Design review of the part built by this model. Coordinates are the model's own, in mm. Coordinates: 2 decimals unless noted, no trailing zeros. Loops run counter-clockwise (first coordinate to the right, second up) from the corner with the lowest first, then second, coordinate; pieces in that order, holes last. Notation, with made-up numbers: (57, 25.25) -> (73, 25.25) arc R20 ccw to (73, 47.25) -> close; hole circle Ø5 at (80, -33). An arc over 180 degrees is marked (long way). Use a Markdown table: item, result. Add a question column.
Q1. Clearance check with flat-ended pins moving along their axes: pin 1 Ø3 at (x, z) = (-33.02, 37.338) entering from +Y; pin 2 Ø1.5 at (x, y) = (172.5, 3.5) entering from +Z; pin 3 Ø1.5 at (x, z) = (-10.5, 17.5) entering from -Y. State where each tip first meets the part, or that it passes through.
Q2. Take a section at B-B on y = 3.85. Count the separate pieces of the cut face and the enclosed holes in it, plus the area to 3 significant figures.
Q3. Take a section at A-A on z = 68.58. Write out the cut boundary in (x, y) (1 decimal), plus the area to 3 significant figures.
Q4. Take a section at C-C on x = 88. Write out the cut boundary in (y, z).
Q5. For probe 1 along X at (y, z) = (3.5, -44.45); probe 2 along Z at (x, y) = (17.78, 2.2); probe 3 along X at (y, z) = (1.35, 70), list the stretches that pass through material, from the lowest coordinate up.
from build123d import *

# Parameters (mm, degrees)
SKETCH1_R               = 22.225
SKETCH1_W               = 373.38
SKETCH1_H               = 127
BOSS_EXTRUDE1_DEPTH     = 5.07492
SKETCH1_5_R             = 6.2865
CUT_EXTRUDE1_DEPTH      = 208.664293845
CUT_EXTRUDE2_DEPTH      = 208.664293845
CUT_EXTRUDE2_DEPTH_BACK = 208.664293845
SKETCH1_7_R             = 3.048
SKETCH1_8_R             = 2.54
SKETCH1_8_R_2           = 3.175
CUT_EXTRUDE3_DEPTH      = 208.664293845


with BuildPart() as part:
    # Sketch1 → Boss-Extrude1 (new body)
    with BuildSketch(Plane(origin=(0, 0, 0), x_dir=(1, 0, 0), z_dir=(0, 1, 0))):
        with Locations((-123.19, -68.58)):
            Circle(SKETCH1_R)
        with Locations((123.19, -68.58)):
            Circle(SKETCH1_R)
        Rectangle(SKETCH1_W, SKETCH1_H)
    extrude(amount=BOSS_EXTRUDE1_DEPTH)

    # Sketch1<5> → Cut-Extrude1 (cut, through all)
    with BuildSketch(Plane(origin=(0, 0, 0), x_dir=(1, 0, 0), z_dir=(0, 1, 0))):
        with Locations(Location((-123.19, -68.58, 0), (0, 0, 90))):
            Circle(SKETCH1_5_R)
        with Locations(Location((123.19, -68.58, 0), (0, 0, 90))):
            Circle(SKETCH1_5_R)
    extrude(amount=CUT_EXTRUDE1_DEPTH, mode=Mode.SUBTRACT)

    # Sketch1<7> → Cut-Extrude2 (cut, two sides: drawn at the far end of the back side and taken through both)
    with BuildSketch(Plane(origin=(0, 0, 0), x_dir=(1, 0, 0), z_dir=(0, 1, 0)).offset(-CUT_EXTRUDE2_DEPTH_BACK)):
        with Locations(Location((-123.19, 44.45, 0), (0, 0, 90))):
            Circle(SKETCH1_7_R)
        with Locations(Location((123.19, 44.45, 0), (0, 0, 90))):
            Circle(SKETCH1_7_R)
    extrude(amount=CUT_EXTRUDE2_DEPTH + CUT_EXTRUDE2_DEPTH_BACK, mode=Mode.SUBTRACT)

    # Sketch1<8> → Cut-Extrude3 (cut, through all)
    with BuildSketch(Plane(origin=(0, 0, 0), x_dir=(1, 0, 0), z_dir=(0, 1, 0))):
        with Locations(Location((-33.02, -37.338, 0), (0, 0, 90))):
            Circle(SKETCH1_8_R)
        with Locations(Location((17.78, -37.338, 0), (0, 0, 90))):
            Circle(SKETCH1_8_R)
        with Locations(Location((0, -54.864, 0), (0, 0, 90))):
            Circle(SKETCH1_8_R_2)
    extrude(amount=CUT_EXTRUDE3_DEPTH, mode=Mode.SUBTRACT)


solid = part.part
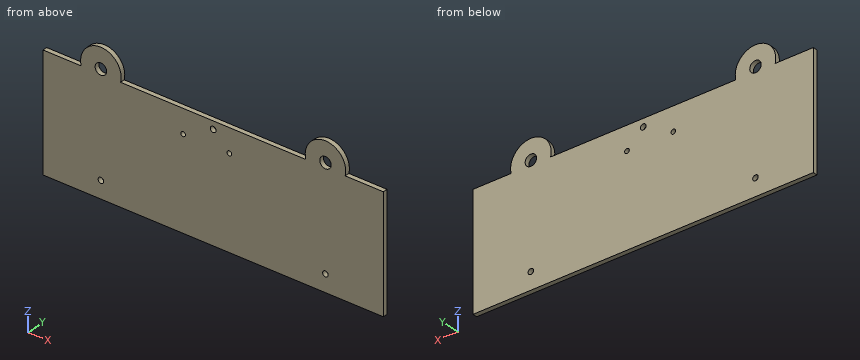
Answer list:
| question | item | result |
|---|---|---|
| 1 | pin 1 | through |
| 1 | pin 2 | z = 63.5 |
| 1 | pin 3 | y = 0 |
| 2 | separate pieces | 1 |
| 2 | enclosed holes | 7 |
| 2 | area | 49,000 mm² |
| 3 | outline | (-145.4, 0) -> (-129.5, 0) -> (-129.5, 5.1) -> (-145.4, 5.1) -> close; (-116.9, 0) -> (-101, 0) -> (-101, 5.1) -> (-116.9, 5.1) -> close; (101, 0) -> (116.9, 0) -> (116.9, 5.1) -> (101, 5.1) -> close; (129.5, 0) -> (145.4, 0) -> (145.4, 5.1) -> (129.5, 5.1) -> close |
| 3 | area | 324 mm² |
| 4 | outline | (0, -63.5) -> (5.07, -63.5) -> (5.07, 63.5) -> (0, 63.5) -> close |
| 5 | probe 1 | -186.69 to -126.24, -120.14 to 120.14, 126.24 to 186.69 |
| 5 | probe 2 | -63.5 to 34.8, 39.88 to 63.5 |
| 5 | probe 3 | -145.37 to -129.31, -117.07 to -101.01, 101.01 to 117.07, 129.31 to 145.37 |
